Could you check a few things on this model? Use its own coordinates, in mm. A direction names the side the tool comes from. Coordinates: 2 decimals unless noted, no trailing zeros. Write each loop counter-clockwise with the first axis right and the second up, starting at its lowest first coordinate (ties: lowest second). Pieces come first, ordered by that corner, then holes. Notation, with made-up numbers: (-24, 6) - (27, 6) arc R20 ccw to (27, 39) - close; hole circle Ø6 at (54.25, 46.5). An arc over 180 degrees is marked (long way). Answer as a JSON object with one key per item and string values. Group by question number.
1) On a 3-axis mill with a long thin cutter (end or side, diameter ignored), from which of +Z, -Z, +X, -X, +Y, -Y can I reach the whole of each face in a straight line? I mean faces 1 (the flat face through (-0.2, -6.5, 0)), 2 (the cylindrical face through (4.57, -7.167, 25.199)). Say none if no direction works.
2) Will these pins go through, and if not, where does the flat tip stop? pin 1 Ø12 at (y, z) = (-4.5, 37.5) entering from -X; pin 2 Ø3 at (y, z) = (-6.5, 37) entering from +X; pin 3 Ø11 at (x, y) = (0, 0) entering from -Z; pin 4 Ø1.5 at (y, z) = (-1.5, 15.5) entering from +X.
3) If we section it at D-D (y = 6.75): Write out the boundary of the cut face in (x, z).
4) If we section it at C-C (z = 36.5): Write out the boundary of the cut face in (x, y), plus the area to 3 significant figures.
5) Please list where these lines run through material, in increasing order: line 1 along Y through (x, z) = (0, 26); line 2 along Z through (x, y) = (-12, 7.25); line 3 along X through (y, z) = (4.25, 43.5).
6) We'd pull the mould along Y, two halves only. Please class faces 3 (the cylindrical face through (-14.985, -0.66, 1.972)), 4 (the flat face through (2, 6, 47)), 5 (the cylindrical face through (-6, 0, 24)): released by +Y, released by -Y, zero draft, split by the parting line, or undercut.
7) If we section it at A-A (y = 0): Write out the boundary of the cut face in (x, z).
Autodesk Inventor part; units mm, degrees
ref_plane "YZ Plane" through (0, 0, 0) normal (1, 0, 0) x (0, 1, 0)
ref_plane "XZ Plane" through (0, 0, 0) normal (0, 1, 0) x (-1, 0, 0)
ref_plane "XY Plane" through (0, 0, 0) normal (0, 0, 1) x (1, 0, 0)
sketch "Boceto1" plane through (0, 0, 0) normal (0, 0, 1) x (1, 0, 0)
  circle A0 centre (0, 0) radius 15
  dimension "d0" = 30
extrude "Extrusión1" add sketch "Boceto1" along normal blind 4
sketch "Boceto2" plane through (0, 0, 4) normal (0, 0, 1) x (1, 0, 0)
  circle A0 centre (0, 0) radius 8.5
  dimension "d3" = 17
extrude "Extrusión2" add sketch "Boceto2" along normal blind 43
sketch "Boceto3" plane through (0, 0, 47) normal (0, 0, 1) x (1, 0, 0)
  circle A0 centre (0, 0) radius 6
  dimension "d6" = 12
extrude "Extrusión3" cut sketch "Boceto3" against normal through all
properties part number "wheel_bush" material "Acero inoxidable"
Here are the results:
{
 "1": {"face 1": "-Z, +X, -X, +Y, -Y", "face 2": "+Z"},
 "2": {"pin 1": "stops at x = -8.5", "pin 2": "stops at x = 6.87", "pin 3": "passes through", "pin 4": "stops at x = 8.47"},
 "3": {"outline": "(-13.4, 0) - (13.4, 0) - (13.4, 4) - (5.17, 4) - (5.17, 47) - (-5.17, 47) - (-5.17, 4) - (-13.4, 4) - close"},
 "4": {"outline": "circle Ø17 at (0, 0); hole circle Ø12 at (0, 0)", "area": "114 mm²"},
 "5": {"line 1": "y = -8.5 to -6, 6 to 8.5", "line 2": "z = 0 to 4", "line 3": "x = -7.36 to -4.24, 4.24 to 7.36"},
 "6": {"face 3": "split by the parting line", "face 4": "zero draft", "face 5": "undercut"},
 "7": {"outline": "(-15, 0) - (-6, 0) - (-6, 47) - (-8.5, 47) - (-8.5, 4) - (-15, 4) - close; (6, 0) - (15, 0) - (15, 4) - (8.5, 4) - (8.5, 47) - (6, 47) - close"}
}
